Can you work these out from the model? Positions are in its coordinate system, mm. Face numbers are marked on the shaded views. Coordinates: 2 decimals unless noted, no trailing zeros. Order: outer loops, then holes, each group sorted by start corner. A loop starts at its lowest first (then second) coordinate and runs counter-clockwise, first axis right, second up. Notation, with made-up numbers: (6.25, -21) -> (16.25, -21) arc R25 ccw to (16.25, -5) -> close; hole circle Ø10 at (-40, 76.25). An arc over 180 degrees is marked (long way). Answer in a Markdown table with one row per item. Add a question column.
1. Imagine slicing it at A-A on y = -1.75. Write out the boundary of the cut face in (x, z), plus the area to 3 significant figures.
2. If I drill on line 1 along X through (y, z) = (-4, 9); line 2 along Z through (x, y) = (23.8, -1.75); line 3 along Y through (x, z) = (6, 16.5), over which ranges is the centre line in solid material (lowest first)? Write a range as [from, to].
3. Imagine slicing it at D-D on z = 8. Write out the boundary of the cut face in (x, y), plus the area to 3 significant figures.
4. Imagine slicing it at B-B on x = -20.5. Write out the boundary of the cut face in (y, z), plus the area to 3 significant figures.
5. Will these pins go through, and if not, where does the flat tip stop? pin 1 (1.2 mm diameter, centred on x = -23.5, y = -1.5, fed in from -Z); pin 2 (1.4 mm diameter, centred on x = -14, y = -10.5, fed in from -Z); pin 3 (1.6 mm diameter, centred on x = 0, z = 29.5, fed in from -Y); pin 4 (1.2 mm diameter, centred on x = -5.5, z = 31, fed in from -Y).
6. Imagine slicing it at C-C on y = -6.5. Write out the boundary of the cut face in (x, z).
7. We'd pull the mould along X, two halves only. Please class the marked faces 1, 2, 3 and 4: pulls with the +X half, pulls with the -X half, needs draft (parallel to the pull), parting line crosses it, or undercut.
from build123d import *

# Parameters (mm, degrees)
BODY_DEPTH                       = 32
BODY_DEPTH_BACK                  = 15
PIVOT_HOLE_DEPTH                 = 42.979905907
PIVOT_HOLE_DEPTH_BACK            = 42.979905907
PIVOT_HOLE_SKETCH_R              = 4.05
OUTSIDE_SHAPE_CUT_OUT_DEPTH      = 42.979905907
OUTSIDE_SHAPE_CUT_OUT_DEPTH_BACK = 42.979905907
OUTSIDE_SHAPE_CUT_OUT_SKETCH_W   = 49
OUTSIDE_SHAPE_CUT_OUT_SKETCH_H   = 22
INSIDE_START                     = 22.05
INSIDE_SHAPE_CUT_OUT_DEPTH       = 44.1
F_3_START                        = -11.75
F_3_M5_SLOTS_DEPTH               = 3.5


with BuildPart() as part:
    # Profile Sketch → Body (new, two sides: drawn at the far end of the back side and taken through both)
    with BuildSketch(Plane.XY.offset(-BODY_DEPTH_BACK)):
        Polygon((-24.5, -11.75), (24.5, -11.75), (24.5, 8.25), (22.05, 8.25), (22.05, -8.25), (-22.05, -8.25), (-22.05, 8.25), (-24.5, 8.25), align=None)
    extrude(amount=BODY_DEPTH + BODY_DEPTH_BACK)

    # Pivot Hole Sketch → Pivot Hole (cut, two sides: drawn at the far end of the back side and taken through both)
    with BuildSketch(Plane(origin=(0, 0, 0), x_dir=(0, 0, -1), z_dir=(1, 0, 0)).offset(-PIVOT_HOLE_DEPTH_BACK)):
        with Locations((0, -1.75)):
            Circle(PIVOT_HOLE_SKETCH_R)
    extrude(amount=PIVOT_HOLE_DEPTH + PIVOT_HOLE_DEPTH_BACK, mode=Mode.SUBTRACT)

    # Outside Shape Cut Out Sketch → Outside Shape Cut Out (cut, two sides: drawn at the far end of the back side and taken through both)
    with BuildSketch(Plane(origin=(0, 0, 0), x_dir=(0, 0, -1), z_dir=(1, 0, 0)).offset(-OUTSIDE_SHAPE_CUT_OUT_DEPTH_BACK)):
        with Locations((-9.5, -2.75)):
            Rectangle(OUTSIDE_SHAPE_CUT_OUT_SKETCH_W, OUTSIDE_SHAPE_CUT_OUT_SKETCH_H)
        with BuildLine():
            Line((-27.649101987, 3.819656009), (-5.267826876, 6.75))
            ThreePointArc((-5.267826876, 6.75), (-3.57284062, 7.589957703), (-1.75, 8.095684334))
            Line((-1.75, 8.095684334), (-1.25, 6.15))
            Line((-1.25, 6.15), (1.25, 6.15))
            Line((1.25, 6.15), (1.75, 8.095684334))
            ThreePointArc((1.75, 8.095684334), (7.071067812, 5.321067812), (9.845684334, 0))
            Line((9.845684334, 0), (7.9, -0.5))
            Line((7.9, -0.5), (7.9, -3))
            Line((7.9, -3), (9.845684334, -3.5))
            ThreePointArc((9.845684334, -3.5), (6.422616289, -9.414854858), (0, -11.75))
            Line((0, -11.75), (-32, -11.75))
            Line((-32, -11.75), (-32, -1.138031619))
            ThreePointArc((-32, -1.138031619), (-30.758025408, 2.160035244), (-27.649101987, 3.819656009))
        make_face(mode=Mode.SUBTRACT)
    extrude(amount=OUTSIDE_SHAPE_CUT_OUT_DEPTH + OUTSIDE_SHAPE_CUT_OUT_DEPTH_BACK, mode=Mode.SUBTRACT)

    # Inside Shape Cut Out Sketch → Inside Shape Cut Out (cut)
    with BuildSketch(Plane(origin=(0, 0, 0), x_dir=(0, 0, -1), z_dir=(1, 0, 0)).offset(INSIDE_START)):
        Polygon((-29, -9.75), (-29, -11.75), (-32, -11.75), (-32, -10.75), (-30.5, -10.75), (-30.5, -9.75), align=None)
        Polygon((-9.5, -8.25), (-5, -10.75), (-5, -11.75), (7.599342077, -11.75), (7.599342077, -8.25), align=None)
    extrude(amount=-INSIDE_SHAPE_CUT_OUT_DEPTH, mode=Mode.SUBTRACT)

    # 3 M5 Slots: read off the stored shape, not the designer's step
    # 3 M5 Slots outline → 3 M5 Slots (cut)
    with BuildSketch(Plane(origin=(0, 0, 0), x_dir=(1, 0, 0), z_dir=(0, 1, 0)).offset(F_3_START)):
        with BuildLine():
            Line((-0.85, -20.65), (0.85, -20.65))
            ThreePointArc((0.85, -20.65), (3.5, -18), (0.85, -15.35))
            Line((0.85, -15.35), (-0.85, -15.35))
            ThreePointArc((-0.85, -15.35), (-3.5, -18), (-0.85, -20.65))
        make_face()
        with BuildLine():
            Line((13.15, -27.65), (14.85, -27.65))
            ThreePointArc((14.85, -27.65), (17.5, -25), (14.85, -22.35))
            Line((14.85, -22.35), (13.15, -22.35))
            ThreePointArc((13.15, -22.35), (10.5, -25), (13.15, -27.65))
        make_face()
        with BuildLine():
            ThreePointArc((-13.15, -27.65), (-10.5, -25), (-13.15, -22.35))
            Line((-13.15, -22.35), (-14.85, -22.35))
            ThreePointArc((-14.85, -22.35), (-17.5, -25), (-14.85, -27.65))
            Line((-14.85, -27.65), (-13.15, -27.65))
        make_face()
    extrude(amount=F_3_M5_SLOTS_DEPTH, mode=Mode.SUBTRACT)

    # 3 M5 Slots 2: loft between two sections, ruled curve by curve
    f_3_m5_slots_2_from = [
        Edge.make_three_point_arc((0.85, -9.6, 20.65), (2.72383297, -9.6, 19.87383297), (3.5, -9.6, 18)),
        Edge.make_three_point_arc((3.5, -9.6, 18), (2.72383297, -9.6, 16.12616703), (0.85, -9.6, 15.35)),
        Edge.make_three_point_arc((-0.85, -9.6, 15.35), (-2.72383297, -9.6, 16.12616703), (-3.5, -9.6, 18)),
        Edge.make_three_point_arc((-3.5, -9.6, 18), (-2.72383297, -9.6, 19.87383297), (-0.85, -9.6, 20.65)),
        Edge.make_line((0.85, -9.6, 15.35), (-0.85, -9.6, 15.35)),
        Edge.make_line((0.85, -9.6, 20.65), (-0.85, -9.6, 20.65)),
    ]
    f_3_m5_slots_2_to = [
        Edge.make_three_point_arc((0.85, -8.25, 22), (3.678427125, -8.25, 20.828427125), (4.85, -8.25, 18)),
        Edge.make_three_point_arc((4.85, -8.25, 18), (3.678427125, -8.25, 15.171572875), (0.85, -8.25, 14)),
        Edge.make_three_point_arc((-0.85, -8.25, 14), (-3.678427125, -8.25, 15.171572875), (-4.85, -8.25, 18)),
        Edge.make_three_point_arc((-4.85, -8.25, 18), (-3.678427125, -8.25, 20.828427125), (-0.85, -8.25, 22)),
        Edge.make_line((0.85, -8.25, 14), (-0.85, -8.25, 14)),
        Edge.make_line((0.85, -8.25, 22), (-0.85, -8.25, 22)),
    ]
    f_3_m5_slots_2 = Solid(Shell([*[Face.make_surface_from_curves(f_3_m5_slots_2_from[k], f_3_m5_slots_2_to[k]) for k in range(6)], Face(Wire(f_3_m5_slots_2_from)), Face(Wire(f_3_m5_slots_2_to))]))
    add(f_3_m5_slots_2, mode=Mode.SUBTRACT)

    # 3 M5 Slots 3: loft between two sections, ruled curve by curve
    f_3_m5_slots_3_from = [
        Edge.make_three_point_arc((14.85, -9.6, 27.65), (16.72383297, -9.6, 26.87383297), (17.5, -9.6, 25)),
        Edge.make_three_point_arc((17.5, -9.6, 25), (16.72383297, -9.6, 23.12616703), (14.85, -9.6, 22.35)),
        Edge.make_three_point_arc((13.15, -9.6, 22.35), (11.27616703, -9.6, 23.12616703), (10.5, -9.6, 25)),
        Edge.make_three_point_arc((10.5, -9.6, 25), (11.27616703, -9.6, 26.87383297), (13.15, -9.6, 27.65)),
        Edge.make_line((14.85, -9.6, 22.35), (13.15, -9.6, 22.35)),
        Edge.make_line((14.85, -9.6, 27.65), (13.15, -9.6, 27.65)),
    ]
    f_3_m5_slots_3_to = [
        Edge.make_three_point_arc((14.85, -8.25, 29), (17.678427125, -8.25, 27.828427125), (18.85, -8.25, 25)),
        Edge.make_three_point_arc((18.85, -8.25, 25), (17.678427125, -8.25, 22.171572875), (14.85, -8.25, 21)),
        Edge.make_three_point_arc((13.15, -8.25, 21), (10.321572875, -8.25, 22.171572875), (9.15, -8.25, 25)),
        Edge.make_three_point_arc((9.15, -8.25, 25), (10.321572875, -8.25, 27.828427125), (13.15, -8.25, 29)),
        Edge.make_line((14.85, -8.25, 21), (13.15, -8.25, 21)),
        Edge.make_line((14.85, -8.25, 29), (13.15, -8.25, 29)),
    ]
    f_3_m5_slots_3 = Solid(Shell([*[Face.make_surface_from_curves(f_3_m5_slots_3_from[k], f_3_m5_slots_3_to[k]) for k in range(6)], Face(Wire(f_3_m5_slots_3_from)), Face(Wire(f_3_m5_slots_3_to))]))
    add(f_3_m5_slots_3, mode=Mode.SUBTRACT)

    # 3 M5 Slots 4: loft between two sections, ruled curve by curve
    f_3_m5_slots_4_from = [
        Edge.make_three_point_arc((-13.15, -9.6, 27.65), (-11.27616703, -9.6, 26.87383297), (-10.5, -9.6, 25)),
        Edge.make_three_point_arc((-10.5, -9.6, 25), (-11.27616703, -9.6, 23.12616703), (-13.15, -9.6, 22.35)),
        Edge.make_three_point_arc((-14.85, -9.6, 22.35), (-16.72383297, -9.6, 23.12616703), (-17.5, -9.6, 25)),
        Edge.make_three_point_arc((-17.5, -9.6, 25), (-16.72383297, -9.6, 26.87383297), (-14.85, -9.6, 27.65)),
        Edge.make_line((-13.15, -9.6, 22.35), (-14.85, -9.6, 22.35)),
        Edge.make_line((-13.15, -9.6, 27.65), (-14.85, -9.6, 27.65)),
    ]
    f_3_m5_slots_4_to = [
        Edge.make_three_point_arc((-13.15, -8.25, 29), (-10.321572875, -8.25, 27.828427125), (-9.15, -8.25, 25)),
        Edge.make_three_point_arc((-9.15, -8.25, 25), (-10.321572875, -8.25, 22.171572875), (-13.15, -8.25, 21)),
        Edge.make_three_point_arc((-14.85, -8.25, 21), (-17.678427125, -8.25, 22.171572875), (-18.85, -8.25, 25)),
        Edge.make_three_point_arc((-18.85, -8.25, 25), (-17.678427125, -8.25, 27.828427125), (-14.85, -8.25, 29)),
        Edge.make_line((-13.15, -8.25, 21), (-14.85, -8.25, 21)),
        Edge.make_line((-13.15, -8.25, 29), (-14.85, -8.25, 29)),
    ]
    f_3_m5_slots_4 = Solid(Shell([*[Face.make_surface_from_curves(f_3_m5_slots_4_from[k], f_3_m5_slots_4_to[k]) for k in range(6)], Face(Wire(f_3_m5_slots_4_from)), Face(Wire(f_3_m5_slots_4_to))]))
    add(f_3_m5_slots_4, mode=Mode.SUBTRACT)


solid = part.part
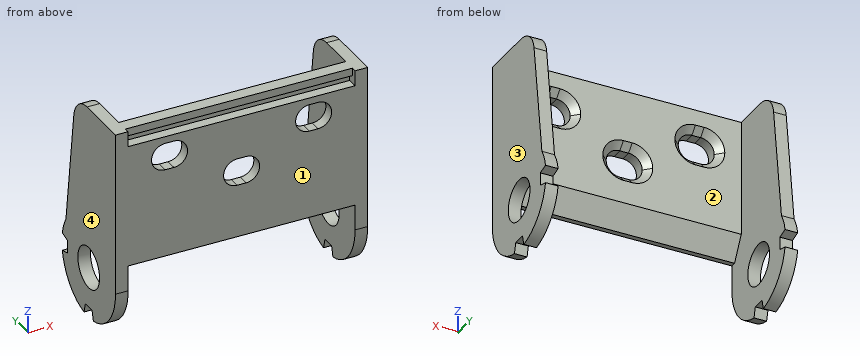
Answers follow:
| question | item | result |
|---|---|---|
| 1 | outline | (-24.5, -7.9) -> (-22.05, -7.9) -> (-22.05, -4.05) -> (-24.5, -4.05) -> close; (-24.5, 4.05) -> (-22.05, 4.05) -> (-22.05, 32) -> (-24.5, 32) -> close; (22.05, -7.9) -> (24.5, -7.9) -> (24.5, -4.05) -> (22.05, -4.05) -> close; (22.05, 4.05) -> (24.5, 4.05) -> (24.5, 32) -> (22.05, 32) -> close |
| 1 | area | 156 mm² |
| 2 | line 1 | x = [-24.5, -22.05], [22.05, 24.5] |
| 2 | line 2 | z = [-7.9, -4.05], [4.05, 32] |
| 2 | line 3 | y = [-11.75, -8.25] |
| 3 | outline | (-24.5, -11.75) -> (24.5, -11.75) -> (24.5, 6.39) -> (22.05, 6.39) -> (22.05, -9.08) -> (-22.05, -9.08) -> (-22.05, 6.39) -> (-24.5, 6.39) -> close |
| 3 | area | 206 mm² |
| 4 | outline | (-11.75, 5) -> (-10.75, 5) -> (-8.25, 9.5) -> (-8.25, 32) -> (-10.75, 32) -> (-10.75, 30.5) -> (-9.75, 30.5) -> (-9.75, 29) -> (-11.75, 29) -> close |
| 4 | area | 84.4 mm² |
| 5 | pin 1 | stops at z = -7.9 |
| 5 | pin 2 | stops at z = 5 |
| 5 | pin 3 | stops at y = -11.75 |
| 5 | pin 4 | stops at y = -10.75 |
| 6 | outline | (-24.5, -8.8) -> (-22.05, -8.8) -> (-22.05, 32) -> (-24.5, 32) -> close; (22.05, -8.8) -> (24.5, -8.8) -> (24.5, 32) -> (22.05, 32) -> close |
| 7 | face 1 | needs draft |
| 7 | face 2 | undercut |
| 7 | face 3 | pulls with the +X half |
| 7 | face 4 | pulls with the -X half |
